Model file for the job. Use its own axes, mm. A direction names the side the tool comes from. Round coordinates to 2 decimals unless told otherwise and drop trailing zeros. Use CSV: the item, a comma, the result in double quotes.
```python
from build123d import *

# Parameters (mm, degrees)
SKETCH004_R       = 6.35
PAD001_DEPTH      = 85
PAD002_DEPTH      = 85
SKETCH016_R       = 5.55
POCKET_DEPTH      = 0.001
POCKET_DEPTH_BACK = 85.001
CHAMFER001_SIZE   = 1


with BuildPart() as part:
    # Sketch004 → Pad001 (new body)
    with BuildSketch(Plane.XZ):
        with Locations((43, 33.25)):
            Circle(SKETCH004_R)
    extrude(amount=PAD001_DEPTH)

    # Sketch017 → Pad002 (join)
    with BuildSketch(Plane.XZ):
        with BuildLine():
            Line((35.113144, 34.25), (50.886856, 34.25))
            ThreePointArc((50.886856, 32.25), (50.95, 33.25), (50.886856, 34.25))
            Line((44, 32.25), (50.886856, 32.25))
            Line((44, 32.25), (44, 25.363144))
            ThreePointArc((42, 25.363144), (43, 25.3), (44, 25.363144))
            Line((42, 32.25), (42, 25.363144))
            Line((35.113144, 32.25), (42, 32.25))
            ThreePointArc((35.113144, 34.25), (35.05, 33.25), (35.113144, 32.25))
        make_face()
    extrude(amount=PAD002_DEPTH)

    # Sketch016 → Pocket (cut, two sides)
    with BuildSketch(Plane.XZ) as pocket_sk:
        with Locations((43, 33.25)):
            Circle(SKETCH016_R)
    extrude(amount=-POCKET_DEPTH, mode=Mode.SUBTRACT)
    extrude(pocket_sk.sketch, amount=POCKET_DEPTH_BACK, mode=Mode.SUBTRACT)

    # Sketch014 (on DatumPlane) → SubtractiveLoft001 section 0
    with BuildSketch(Plane.XY.offset(10)):
        with BuildLine():
            Line((-2, 2), (-2, -87))
            Line((-2, -87), (76.866516, -87))
            Line((76.866516, -38.996654), (76.866516, -87))
            Line((0, -70.790865), (76.866516, -38.996654))
            Line((0, -70.790865), (0, -59.815429))
            ThreePointArc((0, -59.815429), (18.580156, -58.2705), (36.65, -53.678146))
            Line((36.65, -53.678146), (36.65, -51.378146))
            Line((36.65, -51.378146), (35.967157, -50.695303))
            ThreePointArc((35.967157, -50.129618), (35.85, -50.41246), (35.967157, -50.695303))
            Line((35.967157, -50.129618), (36.65, -49.446775))
            Line((36.65, -49.446775), (49.35, -44.182166))
            Line((50.032843, -44.865009), (49.35, -44.182166))
            ThreePointArc((50.032843, -45.430695), (50.15, -45.147852), (50.032843, -44.865009))
            Line((49.35, -46.113537), (50.032843, -45.430695))
            Line((49.35, -48.413537), (49.35, -46.113537))
            ThreePointArc((49.35, -48.413537), (64.17388, -39.716528), (77.5, -28.862961))
            Line((77.5, 2), (77.5, -28.862961))
            Line((-2, 2), (77.5, 2))
        make_face()
    # Sketch015 (on DatumPlane) → SubtractiveLoft001 section 1
    with BuildSketch(Plane.XY.offset(42)):
        with BuildLine():
            Line((-2, 2), (-2, -87))
            Line((-2, -87), (63.5, -87))
            Line((63.5, -87), (63.5, -27.765276))
            Line((0, -58.577105), (63.5, -27.765276))
            Line((0, -58.577105), (0, -45.815429))
            ThreePointArc((0, -45.815429), (18.663063, -44.031199), (36.65, -38.743146))
            Line((36.65, -38.743146), (36.65, -36.543146))
            Line((36.65, -36.543146), (35.967157, -35.860304))
            ThreePointArc((35.967157, -35.294618), (35.85, -35.577461), (35.967157, -35.860304))
            Line((35.967157, -35.294618), (36.65, -34.611775))
            Line((49.35, -28.429747), (36.65, -34.611775))
            Line((50.032843, -29.11259), (49.35, -28.429747))
            ThreePointArc((50.032843, -29.678275), (50.15, -29.395433), (50.032843, -29.11259))
            Line((49.35, -30.361118), (50.032843, -29.678275))
            Line((49.35, -30.361118), (49.35, -32.561118))
            ThreePointArc((49.35, -32.561118), (56.643736, -27.899157), (63.5, -22.614831))
            Line((63.5, 2), (63.5, -22.614831))
            Line((63.5, 2), (-2, 2))
        make_face()
    loft(mode=Mode.SUBTRACT)

    # Chamfer001
    chamfer001_edges = [part.edges().sort_by_distance(p)[0] for p in [
        (35.050008, -45.689757, 33.261359),
        (43.011121, -45.833884, 25.300008),
        (50.934027, -38.597846, 32.746296),
    ]]
    chamfer(chamfer001_edges, length=CHAMFER001_SIZE)


solid = part.part
```
Q1. Mould opens along X. For faces 1 (the cylindrical face through (48.127, -38.73, 31.124)), 2 (the flat face through (42, -42, 26)), 3 (the flat face through (50.4, -36.1, 34.25)) say: +X half, -X half, draft (parallel to the pull), parting line (faces both ways), or undercut.
From the geometry:
face 1,"undercut"
face 2,"-X half"
face 3,"draft"
Q2. Which spindle directions (+Z, -Z, +X, -X, +Y, -Y) get a long thin tool onto all of the face, cutting with end or side? Do faces 4 (the flat face through (36, -44, 32.25)), 5 (the flat face through (36, -43, 34.25)), 6 (the flat face through (50.25, -37.09, 32.25)), 7 (the cylindrical face through (43.1, -36.4, 39.6)), 8 (the cylindrical face through (50.95, -36.62, 33.24)). Say none if no direction does.
From the geometry:
face 4,"-Z, -X, +Y, -Y"
face 5,"+Z, -X, +Y, -Y"
face 6,"-Z, +X, +Y, -Y"
face 7,"+Z, +Y, -Y"
face 8,"+X, +Y, -Y"
Q3. Probe line 1 along X through (y, z) = (-41.5, 33.25); line 2 along Z through (x, y) = (38, -42); line 3 along X through (y, z) = (-36.75, 33.25). List the from-to ranges inside material, lowest first.
From the geometry:
line 1,"x = 36.65 to 37.45"
line 2,"z = 29.34 to 30.84, 35.66 to 37.16"
line 3,"x = 48.55 to 49.35, 49.62 to 50.95"
Q4. Pin check, flat tips, straight feed: pin 1 (1 mm diameter, centred on x = 40.5, z = 27.5, fed in from -Y); pin 2 (4 mm diameter, centred on y = -41, z = 32, fed in from +X); pin 3 (6 mm diameter, centred on x = 42, z = 35.5, fed in from +Y) (3 decimals); pin 4 (1.5 mm diameter, centred on y = -42, z = 35.5, fed in from -X). Stop position of each tip, or through.
From the geometry:
pin 1,"stops at y = -46.06"
pin 2,"stops at x = 50.1"
pin 3,"passes through"
pin 4,"stops at x = 36.83"
